The model under review builds one solid part; all positions refer to its coordinate system, in mm. A direction names the side the tool comes from. Coordinates: 2 decimals unless noted, no trailing zeros. Order: outer loops, then holes, each group sorted by start corner. A loop starts at its lowest first (then second) coordinate and runs counter-clockwise, first axis right, second up. Notation, with made-up numbers: M -6,42 L 26,42 A21 ccw 26,62 Z; hole C -22.5,68 d3. An arc over 180 degrees is marked long. One line per item, written item: value.
Autodesk Inventor part; units mm, degrees
ref_plane "YZ Plane" through (0, 0, 0) normal (1, 0, 0) x (0, 1, 0)
ref_plane "XZ Plane" through (0, 0, 0) normal (0, 1, 0) x (-1, 0, 0)
ref_plane "XY Plane" through (0, 0, 0) normal (0, 0, 1) x (1, 0, 0)
sketch "Sketch1" plane through (0, 0, 0) normal (0, 1, 0) x (-1, 0, 0)
  line L0 (0, 0) -> (-17, 0)
  line L1 (-17, 0) -> (-17, -26)
  line L2 (-17, -26) -> (0, -26)
  line L3 (0, -26) -> (0, 0)
  dimension "d0" = 26
  dimension "d1" = 17
extrude "Extrusion1" add sketch "Sketch1" along normal blind 45
fillet "Fillet1" radius 2 4 edges at (0, 22.5, -26) (0, 22.5, 0) (17, 22.5, -26) (17, 22.5, 0)
sketch "Sketch2" plane through (0, 45, 0) normal (0, 1, 0) x (1, 0, 0)
  circle A0 centre (8.5, 19.5) radius 2.875
  line L0 (15, 26) -> (2, 26)
  circle A1 centre (8.5, 6.5) radius 4.5
  line L1 (0, 24) -> (0, 2)
  line L2 (2, 0) -> (15, 0)
  point P0 (0, 0)
  dimension "d5" = 5.75
  dimension "d6" = 6.5
  dimension "d7" = 9
  dimension "d8" = 8.5
  dimension "d9" = 8.5
  dimension "d10" = 6.5
extrude "Extrusion2" add sketch "Sketch2" along normal blind 3.3
shell "Shell1" thickness 1 removed faces 2 at (7.7246, 48.3, -18.7113) at (10.0336, 48.3, -5.5053)
properties part number "battery model"
(1) For L1, parallel to Z at x = 8.5, y = 46.95 (3 decimals); L2, parallel to Z at x = 14, y = 12; L3, parallel to Z at x = 8.5, y = 44.9 (3 decimals), list the stretches that pass through material, from the lowest coordinate up.
Geometry results:
L1: z = -22.375 to -21.375, -17.625 to -16.625, -11 to -10, -3 to -2
L2: z = -26 to -25, -1 to 0
L3: z = -26 to -21.375, -17.625 to -10, -3 to 0
(2) Tool access review of faces 4 (the cylindrical face through (7.877, 46.627, -22.307)), 5 (the cylindrical face through (1.301, 22.801, -24.715)), 6 (the flat face through (8, 22, 0)): name each direction out of +Z, -Z, +X, -X, +Y, -Y from which nothing blocks a thin tool from reaching the whole face with its end or side.
Geometry results:
face 4: +Y
face 5: none
face 6: +Z, +X, -X, +Y, -Y
(3) We need section D-D, the plane x = 14.5. State the section outline as (y, z) points.
Geometry results:
outline: M 0,-26 L 45,-26 L 45,0 L 0,0 Z; hole M 1,-25 L 44,-25 L 44,-1 L 1,-1 Z
(4) Insertion check: pin 1 Ø1 at (x, z) = (8, -6.5) entering from +Y. The pin has a flat end and moves straight along its axis. Give the tip position at first contact, or say it passes through.
Geometry results:
pin 1: stops at y = 1
(5) We need section B-B, the plane z = -15.75. State the section outline as (x, y) points, plus the area to 3 significant figures.
Geometry results:
outline: M 0,0 L 17,0 L 17,45 L 0,45 Z; hole M 1,1 L 16,1 L 16,44 L 1,44 Z
area: 120 mm2
(6) We need section A-A, the plane x = 8.5. State the section outline as (y, z) points (3 decimals).
Geometry results:
outline: M 0,-26 L 45,-26 L 45,-22.375 L 48.3,-22.375 L 48.3,-21.375 L 44,-21.375 L 44,-25 L 1,-25 L 1,-1 L 44,-1 L 44,-3 L 48.3,-3 L 48.3,-2 L 45,-2 L 45,0 L 0,0 Z; M 44,-17.625 L 48.3,-17.625 L 48.3,-16.625 L 45,-16.625 L 45,-11 L 48.3,-11 L 48.3,-10 L 44,-10 Z
(7) We need section C-C, the plane y = 14. State the section outline as (x, z) points.
Geometry results:
outline: M 0,-24 A2 ccw 2,-26 L 15,-26 A2 ccw 17,-24 L 17,-2 A2 ccw 15,0 L 2,0 A2 ccw 0,-2 Z; hole M 1,-24 A1 ccw 2,-25 L 15,-25 A1 ccw 16,-24 L 16,-2 A1 ccw 15,-1 L 2,-1 A1 ccw 1,-2 Z
(8) Mouldability with a two-part tool opening along Z and no side actions: class faces 1 (the cylindrical face through (16.4, 22.82, -0.57)), 2 (the cylindrical face through (1.285, 22.801, -1.301)), 3 (the flat face through (9, 0, -13)) as +Z half, -Z half, draft (parallel to the pull), parting line (faces both ways), or undercut.
Geometry results:
face 1: +Z half
face 2: undercut
face 3: draft
